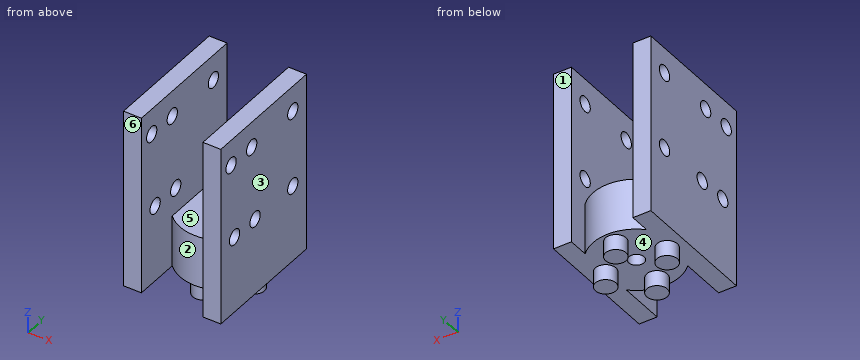
```python
from build123d import *

# Parameters (mm, degrees)
SKETCH_R          = 8.5
SKETCH_R_2        = 1.5
PAD_DEPTH         = 10
SKETCH001_R       = 2
PAD001_DEPTH      = 3
SKETCH002_W       = 3.5
SKETCH002_H       = 25
PAD002_DEPTH      = 25
PAD002_DEPTH_BACK = 10
SKETCH003_R       = 1.5
POCKET_DEPTH      = 19.001


with BuildPart() as part:
    # Sketch → Pad (new body)
    with BuildSketch(Plane.XY):
        Circle(SKETCH_R)
        Circle(SKETCH_R_2, mode=Mode.SUBTRACT)
    extrude(amount=PAD_DEPTH)

    # Sketch001 → Pad001 (new body)
    with BuildSketch(Plane(origin=(0, 0, 0), x_dir=(1, 0, 0), z_dir=(0, 0, -1))):
        with Locations((0, -6)):
            Circle(SKETCH001_R)
        with Locations((6, 0)):
            Circle(SKETCH001_R)
        with Locations((0, 6)):
            Circle(SKETCH001_R)
        with Locations((-6, 0)):
            Circle(SKETCH001_R)
    extrude(amount=PAD001_DEPTH)

    # Sketch002 → Pad002 (new body, two sides)
    with BuildSketch(Plane.XY.offset(10)) as pad002_sk:
        with Locations((-7.75, -2.5)):
            Rectangle(SKETCH002_W, SKETCH002_H)
        with Locations((7.75, -2.5)):
            Rectangle(SKETCH002_W, SKETCH002_H)
    extrude(amount=PAD002_DEPTH)
    extrude(pad002_sk.sketch, amount=-PAD002_DEPTH_BACK)

    # Sketch003 → Pocket (cut, through all)
    with BuildSketch(Plane.YZ.offset(9.5)):
        with Locations((-11, 15)):
            Circle(SKETCH003_R)
        with Locations((-5, 15)):
            Circle(SKETCH003_R)
        with Locations((-12, 30)):
            Circle(SKETCH003_R)
        with Locations((-6, 30)):
            Circle(SKETCH003_R)
        with Locations((6, 30)):
            Circle(SKETCH003_R)
        with Locations((6, 15)):
            Circle(SKETCH003_R)
    extrude(amount=-POCKET_DEPTH, mode=Mode.SUBTRACT)


solid = part.part
```
Source: CAD feature listing. Evaluate the final solid. Frame: model axes, mm. Face numbers are marked on the shaded views. A direction names the side the tool comes from. Round coordinates to 2 decimals unless told otherwise and drop trailing zeros. Loops run counter-clockwise (first coordinate to the right, second up) from the corner with the lowest first, then second, coordinate; pieces in that order, holes last. Notation, with made-up numbers: M 15,63.25 L 54,63.25 A19 ccw 54,87.25 Z; hole C 69.25,-16 d3. An arc over 180 degrees is marked long. Put each result on its own line as item: value.
(1) Section B-B, the plane x = 0. Return loops of the section in (y, z).
Solutions:
outline: M -8.5,0 L -8,0 L -8,-3 L -4,-3 L -4,0 L -1.5,0 L -1.5,10 L -8.5,10 Z; M 1.5,0 L 4,0 L 4,-3 L 8,-3 L 8,0 L 8.5,0 L 8.5,10 L 1.5,10 Z
(2) Section D-D, the plane z = 22.5. Return loops of the section in (x, y).
Solutions:
outline: M -9.5,-15 L -6,-15 L -6,10 L -9.5,10 Z; M 6,-15 L 9.5,-15 L 9.5,10 L 6,10 Z
(3) Ray query, line 1 (X direction, y = 1, z = 18); line 2 (Y direction, x = 7.25, z = 15.5); line 3 (Z direction, x = -8.5, y = -11). Return the intervals inside material, ascending. Write a range as [from, to].
Solutions:
line 1: [-9.5, -6], [6, 9.5]
line 2: [-15, -12.41], [-9.59, -6.41], [-3.59, 4.59], [7.41, 10]
line 3: [0, 13.5], [16.5, 28.88], [31.12, 35]
(4) Section C-C, the plane z = 30. State how many separate pieces and enclosed holes the cut face has, and give its area (3 significant figures).
Solutions:
separate pieces: 8
enclosed holes: 0
area: 112 mm²
(5) First-contact query: pin 1 (6 mm diameter, centred on x = -2.5, z = 9, fed in from -Y); pin 2 (1.8 mm diameter, centred on y = 6, z = 30, fed in from -X); pin 3 (4 mm diameter, centred on x = 0, y = 0, fed in from +Z). Flat tips, straight axial feed; report the tip coordinate or a pass-through.
Solutions:
pin 1: y = -8.5
pin 2: through
pin 3: z = 10
(6) Pull-direction query (X, two-part tool) for the marked faces 1, 2 and 3; classes: released by +X, released by -X, zero draft, split by the parting line, or undercut.
Solutions:
face 1: zero draft
face 2: undercut
face 3: released by +X
(7) Section A-A, the plane y = 0. Return loops of the section in (x, z), and give its area (3 significant figures).
Solutions:
outline: M -9.5,0 L -8,0 L -8,-3 L -4,-3 L -4,0 L -1.5,0 L -1.5,10 L -6,10 L -6,35 L -9.5,35 Z; M 1.5,0 L 4,0 L 4,-3 L 8,-3 L 8,0 L 9.5,0 L 9.5,35 L 6,35 L 6,10 L 1.5,10 Z
area: 359 mm²
(8) Access query for the marked faces 4, 5 and 6. Directions: +Z, -Z, +X, -X, +Y, -Y. A direction counts if a zero-diameter tool reaches every point of the face in a straight line with its end or side. Return the directions, or none.
Solutions:
face 4: -Z
face 5: +Z, +Y, -Y
face 6: +Z, -Z, +X, -X, -Y
